Check sheet for the modelled part. Datum: model origin and axes. Units: mm. A direction names the side the tool comes from. Round coordinates to 2 decimals unless told otherwise and drop trailing zeros. Order: outer loops, then holes, each group sorted by start corner. A loop starts at its lowest first (then second) coordinate and runs counter-clockwise, first axis right, second up. Notation, with made-up numbers: M 52,60 L 73,60 A31 ccw 73,94 Z; hole C 42.5,-32.75 d2. An arc over 180 degrees is marked long. One line per item, written item: value. Start each with the question number.
(1) Depth check by flat-ended pin: pin 1 Ø12 at (x, z) = (13.5, -10.5) entering from +Y; pin 2 Ø4 at (x, z) = (48.5, 27) entering from +Y. Enter the tip coordinate at first touch or a pass-through.
(2) Cross-section at A-A, the plane x = 47.6. Enter the section's corners in (y, z).
(3) Thickness scan on L1, parallel to Z at x = -47.6, y = 2.5; L2, parallel to Z at x = 47.6, y = 4.75; L3, parallel to Z at x = -7.5, y = 19.75. Record the ranges inside material, lowest first.
(4) Cross-section at B-B, the plane z = 27.6. Enter the section's corners in (x, y), and give its area (3 significant figures).
(5) Cross-section at D-D, the plane y = 18. Enter the section's corners in (x, z), and give its area (3 significant figures).
(6) Access from +Z, -Z, +X, -X, +Y, -Y to the whole of each face (thin tool, end or side, straight path). Record for faces 3 (the face through (-1, 14, 33)), 4 (the face through (-13, 2, -14)), 5 (the face through (-54, 5, 20)).
(7) Release check for a two-part mould opening along Y. For faces 1 (the face through (54, 5, 20)), 2 (the face through (8, 2, -18)) record: released by +Y, released by -Y, zero draft, split by the parting line, or undercut.
(8) Cross-section at C-C, the plane x = -27. Enter the section's corners in (y, z), and give its area (3 significant figures).
from build123d import *

# Parameters (mm, degrees)
SKETCH1_W                = 106
SKETCH1_H                = 66
SKETCH1_R                = 2
BOSS_EXTRUDE1_DEPTH      = 3
SKETCH2_W                = 112
SKETCH2_H                = 72
SKETCH2_W_2              = 106
SKETCH2_H_2              = 66
BOSS_EXTRUDE2_DEPTH      = 20
BOSS_EXTRUDE2_DEPTH_BACK = 3
SKETCH4_W                = 109
SKETCH4_H                = 69
SKETCH4_W_2              = 106
SKETCH4_H_2              = 66
BOSS_EXTRUDE3_DEPTH      = 2
CUT_EXTRUDE1_DEPTH       = 4
SKETCH6_R                = 4
SKETCH6_R_2              = 2
BOSS_EXTRUDE4_DEPTH      = 5
SKETCH7_W                = 7
SKETCH7_H                = 7
CUT_EXTRUDE2_DEPTH       = 4


with BuildPart() as part:
    # Sketch1 → Boss-Extrude1 (new body)
    with BuildSketch(Plane(origin=(0, 0, 0), x_dir=(1, 0, 0), z_dir=(0, 1, 0))):
        Rectangle(SKETCH1_W, SKETCH1_H)
        with Locations((-47.6, 27.6)):
            Circle(SKETCH1_R, mode=Mode.SUBTRACT)
        with Locations((47.6, 27.6)):
            Circle(SKETCH1_R, mode=Mode.SUBTRACT)
        with Locations((47.6, -27.6)):
            Circle(SKETCH1_R, mode=Mode.SUBTRACT)
        with Locations((-47.6, -27.6)):
            Circle(SKETCH1_R, mode=Mode.SUBTRACT)
    extrude(amount=BOSS_EXTRUDE1_DEPTH)

    # Sketch2 → Boss-Extrude2 (add, two sides)
    with BuildSketch(Plane(origin=(0, 3, 0), x_dir=(1, 0, 0), z_dir=(0, 1, 0))) as boss_extrude2_sk:
        Rectangle(SKETCH2_W, SKETCH2_H)
        Rectangle(SKETCH2_W_2, SKETCH2_H_2, mode=Mode.SUBTRACT)
    extrude(amount=BOSS_EXTRUDE2_DEPTH)
    extrude(boss_extrude2_sk.sketch, amount=-BOSS_EXTRUDE2_DEPTH_BACK)

    # Sketch4 → Boss-Extrude3 (add)
    with BuildSketch(Plane(origin=(0, 23, 0), x_dir=(1, 0, 0), z_dir=(0, 1, 0))):
        Rectangle(SKETCH4_W, SKETCH4_H)
        Rectangle(SKETCH4_W_2, SKETCH4_H_2, mode=Mode.SUBTRACT)
    extrude(amount=BOSS_EXTRUDE3_DEPTH)

    # Sketch5 → Cut-Extrude1 (cut, through all)
    with BuildSketch(Plane.ZY.offset(-53)):
        with BuildLine():
            Line((5, 3), (10, 3))
            Line((10, 3), (10, 6.5))
            ThreePointArc((10, 6.5), (9.560660172, 7.560660172), (8.5, 8))
            Line((8.5, 8), (6.5, 8))
            ThreePointArc((6.5, 8), (5.439339828, 7.560660172), (5, 6.5))
            Line((5, 6.5), (5, 3))
        make_face()
        with BuildLine():
            Line((20, 3), (25, 3))
            Line((25, 3), (25, 6.5))
            ThreePointArc((25, 6.5), (24.560660172, 7.560660172), (23.5, 8))
            Line((23.5, 8), (21.5, 8))
            ThreePointArc((21.5, 8), (20.439339828, 7.560660172), (20, 6.5))
            Line((20, 6.5), (20, 3))
        make_face()
    cut_extrude1 = extrude(amount=-CUT_EXTRUDE1_DEPTH, mode=Mode.SUBTRACT)

    # Sketch6 → Boss-Extrude4 (add)
    with BuildSketch(Plane(origin=(0, 3, 0), x_dir=(1, 0, 0), z_dir=(0, 1, 0))):
        with Locations((-47.6, 27.6)):
            Circle(SKETCH6_R)
        with Locations((-47.6, 27.6)):
            Circle(SKETCH6_R_2, mode=Mode.SUBTRACT)
        with Locations((47.6, 27.6)):
            Circle(SKETCH6_R)
        with Locations((47.6, 27.6)):
            Circle(SKETCH6_R_2, mode=Mode.SUBTRACT)
        with Locations((47.6, -27.6)):
            Circle(SKETCH6_R)
        with Locations((47.6, -27.6)):
            Circle(SKETCH6_R_2, mode=Mode.SUBTRACT)
        with Locations((-47.6, -27.6)):
            Circle(SKETCH6_R)
        with Locations((-47.6, -27.6)):
            Circle(SKETCH6_R_2, mode=Mode.SUBTRACT)
    extrude(amount=BOSS_EXTRUDE4_DEPTH)

    # Sketch7 → Cut-Extrude2 (cut, through all)
    with BuildSketch(Plane(origin=(0, 3, 0), x_dir=(1, 0, 0), z_dir=(0, 1, 0))):
        with Locations((-9.5, 14.5)):
            Rectangle(SKETCH7_W, SKETCH7_H)
        with Locations((-27.5, 14.5)):
            Rectangle(SKETCH7_W, SKETCH7_H)
        with Locations((8.5, 14.5)):
            Rectangle(SKETCH7_W, SKETCH7_H)
        with Locations((26.5, 14.5)):
            Rectangle(SKETCH7_W, SKETCH7_H)
        with Locations((-9.5, -0.5)):
            Rectangle(SKETCH7_W, SKETCH7_H)
        with Locations((8.5, -0.5)):
            Rectangle(SKETCH7_W, SKETCH7_H)
        with Locations((26.5, -0.5)):
            Rectangle(SKETCH7_W, SKETCH7_H)
        with Locations((-9.5, -15.5)):
            Rectangle(SKETCH7_W, SKETCH7_H)
        with Locations((8.5, -15.5)):
            Rectangle(SKETCH7_W, SKETCH7_H)
        with Locations((26.5, -15.5)):
            Rectangle(SKETCH7_W, SKETCH7_H)
        with Locations((-27.5, -0.5)):
            Rectangle(SKETCH7_W, SKETCH7_H)
        with Locations((-27.5, -15.5)):
            Rectangle(SKETCH7_W, SKETCH7_H)
    extrude(amount=-CUT_EXTRUDE2_DEPTH, mode=Mode.SUBTRACT)

    # Mirror1: Cut-Extrude1 across plane
    add(cut_extrude1.mirror(Plane(origin=(0, 0, 0), x_dir=(0, 0, 1), z_dir=(1, 0, 0))), mode=Mode.SUBTRACT)


solid = part.part
Values found:
1. pin 1: y = 3
1. pin 2: y = 8
2. outline: M 0,-36 L 23,-36 L 23,-34.5 L 25,-34.5 L 25,-33 L 3,-33 L 3,-31.6 L 8,-31.6 L 8,-29.6 L 0,-29.6 Z; M 0,-25.6 L 8,-25.6 L 8,-23.6 L 3,-23.6 L 3,23.6 L 8,23.6 L 8,25.6 L 0,25.6 Z; M 0,29.6 L 8,29.6 L 8,31.6 L 3,31.6 L 3,33 L 25,33 L 25,34.5 L 23,34.5 L 23,36 L 0,36 Z
3. L1: -36 to -29.6, -25.6 to 25.6, 29.6 to 36
3. L2: -36 to -33, -31.6 to -29.6, -25.6 to -23.6, 23.6 to 25.6, 29.6 to 31.6, 33 to 36
3. L3: -36 to -33, 33 to 36
4. outline: M -56,0 L -49.6,0 L -49.6,8 L -51.6,8 L -51.6,3 L -53,3 L -53,25 L -54.5,25 L -54.5,23 L -56,23 Z; M -45.6,0 L 45.6,0 L 45.6,8 L 43.6,8 L 43.6,3 L -43.6,3 L -43.6,8 L -45.6,8 Z; M 49.6,0 L 56,0 L 56,23 L 54.5,23 L 54.5,25 L 53,25 L 53,3 L 51.6,3 L 51.6,8 L 49.6,8 Z
4. area: 478 mm^2
5. outline: M -56,-36 L 56,-36 L 56,36 L -56,36 Z; hole M -53,-33 L 53,-33 L 53,33 L -53,33 Z
5. area: 1,070 mm^2
6. face 3: +Y
6. face 4: +Y, -Y
6. face 5: +X, -X
7. face 1: undercut
7. face 2: zero draft
8. outline: M 0,-36 L 23,-36 L 23,-34.5 L 25,-34.5 L 25,-33 L 3,-33 L 3,-18 L 0,-18 Z; M 0,-11 L 3,-11 L 3,-3 L 0,-3 Z; M 0,4 L 3,4 L 3,12 L 0,12 Z; M 0,19 L 3,19 L 3,33 L 25,33 L 25,34.5 L 23,34.5 L 23,36 L 0,36 Z
8. area: 279 mm^2
